Source: CAD feature listing. Evaluate the final solid. Frame: model axes, mm. A direction names the side the tool comes from. Round coordinates to 2 decimals unless told otherwise and drop trailing zeros. Loops run counter-clockwise (first coordinate to the right, second up) from the corner with the lowest first, then second, coordinate; pieces in that order, holes last. Notation, with made-up numbers: M 63,83 L 74,83 A8 cw 74,96 Z; hole C 0,10.5 d9. An arc over 180 degrees is marked long. One line per item, written item: value.
from build123d import *

# Parameters (mm, degrees)
SKETCH_1_R          = 31.5
EXTRUDE_1_DEPTH     = 8
SKETCH_1_3_R        = 3.25
CUT_EXTRUDE_1_DEPTH = 8
SKETCH_1_4_R        = 17
CUT_EXTRUDE_2_DEPTH = 6
EXTRUDE_2_DEPTH     = 4
SKETCH_4_W          = 50
SKETCH_4_H          = 8.5
EXTRUDE_3_DEPTH     = 95
SKETCH_5_R          = 3.1
CUT_EXTRUDE_3_DEPTH = 10
SKETCH_5_3_R        = 6.75
SKETCH_5_3_R_2      = 3.1
CUT_EXTRUDE_4_DEPTH = 4.3
EXTRUDE_4_DEPTH     = 8
SKETCH_1_8_R        = 17
CUT_EXTRUDE_5_DEPTH = 8


with BuildPart() as part:
    # Sketch 1 → Extrude 1 (new body)
    with BuildSketch(Plane.XY):
        Circle(SKETCH_1_R)
    extrude(amount=EXTRUDE_1_DEPTH)

    # Sketch 1_3 → Cut-Extrude 1 (cut)
    with BuildSketch(Plane.XY):
        with Locations((0, 25)):
            Circle(SKETCH_1_3_R)
        with Locations((-25, 0)):
            Circle(SKETCH_1_3_R)
        with Locations((25, 0)):
            Circle(SKETCH_1_3_R)
        with Locations((0, -25)):
            Circle(SKETCH_1_3_R)
    extrude(amount=CUT_EXTRUDE_1_DEPTH, mode=Mode.SUBTRACT)

    # Sketch 1_4 → Cut-Extrude 2 (cut)
    with BuildSketch(Plane.XY):
        Circle(SKETCH_1_4_R)
    extrude(amount=CUT_EXTRUDE_2_DEPTH, mode=Mode.SUBTRACT)

    # Sketch 1_5 → Extrude 2 (add)
    with BuildSketch(Plane.XY):
        with BuildLine():
            Line((25, 69.163767897), (17.863752341, 69.163767897))
            Line((17.863752341, 69.163767897), (-25, 69.163767897))
            Line((-25, 69.163767897), (-25, 28.735067362))
            Line((-25, 28.735067362), (-25, 19.163767897))
            ThreePointArc((-25, 19.163767897), (0, 31.5), (25, 19.163767897))
            Line((25, 19.163767897), (25, 69.163767897))
        make_face()
    extrude(amount=EXTRUDE_2_DEPTH)

    # Sketch 4 → Extrude 3 (add)
    with BuildSketch(Plane.XY.offset(4)):
        with Locations((0, 64.913767897)):
            Rectangle(SKETCH_4_W, SKETCH_4_H)
    extrude(amount=EXTRUDE_3_DEPTH)

    # Sketch 5 → Cut-Extrude 3 (cut)
    with BuildSketch(Plane.XZ.offset(-60.663767897)):
        with Locations(Location((0.088398714, 90, 0), (0, 0, 270))):
            Circle(SKETCH_5_R)
        with Locations(Location((0.088398714, 20, 0), (0, 0, 270))):
            Circle(SKETCH_5_R)
        with Locations(Location((0.088398714, 43.333, 0), (0, 0, 270))):
            Circle(SKETCH_5_R)
        with Locations(Location((0.088398714, 66.66667, 0), (0, 0, 270))):
            Circle(SKETCH_5_R)
    extrude(amount=-CUT_EXTRUDE_3_DEPTH, mode=Mode.SUBTRACT)

    # Sketch 5_3 → Cut-Extrude 4 (cut)
    # profile 1 of 4: a face of its own
    with BuildSketch(Plane.XZ.offset(-60.663767897)):
        with Locations(Location((0.088398714, 66.66667, 0), (0, 0, 270))):
            Circle(SKETCH_5_3_R)
        with Locations(Location((0.088398714, 66.66667, 0), (0, 0, 270))):
            Circle(SKETCH_5_3_R_2, mode=Mode.SUBTRACT)
    # profile 2 of 4: a face of its own
    with BuildSketch(Plane.XZ.offset(-60.663767897)):
        with Locations(Location((0.088398714, 43.333, 0), (0, 0, 270))):
            Circle(SKETCH_5_3_R)
        with Locations(Location((0.088398714, 43.333, 0), (0, 0, 270))):
            Circle(SKETCH_5_3_R_2, mode=Mode.SUBTRACT)
    # profile 3 of 4: a face of its own
    with BuildSketch(Plane.XZ.offset(-60.663767897)):
        with Locations(Location((0.088398714, 20, 0), (0, 0, 270))):
            Circle(SKETCH_5_3_R)
        with Locations(Location((0.088398714, 20, 0), (0, 0, 270))):
            Circle(SKETCH_5_3_R_2, mode=Mode.SUBTRACT)
    # profile 4 of 4: a face of its own
    with BuildSketch(Plane.XZ.offset(-60.663767897)):
        with Locations(Location((0.088398714, 90, 0), (0, 0, 270))):
            Circle(SKETCH_5_3_R)
    extrude(amount=-CUT_EXTRUDE_4_DEPTH, mode=Mode.SUBTRACT)

    # Sketch 1_7 → Extrude 4 (add)
    with BuildSketch(Plane.XY):
        with BuildLine():
            Line((25, 69.163767897), (17.863752341, 69.163767897))
            Line((17.863752341, 69.163767897), (-25, 69.163767897))
            Line((-25, 69.163767897), (-25, 28.735067362))
            Line((-25, 28.735067362), (-25, 19.163767897))
            ThreePointArc((-25, 19.163767897), (0, 31.5), (25, 19.163767897))
            Line((25, 19.163767897), (25, 69.163767897))
        make_face()
    extrude(amount=EXTRUDE_4_DEPTH)

    # Sketch 1_8 → Cut-Extrude 5 (cut)
    with BuildSketch(Plane.XY):
        Circle(SKETCH_1_8_R)
    extrude(amount=CUT_EXTRUDE_5_DEPTH, mode=Mode.SUBTRACT)


solid = part.part
1. Reachability of faces 1 (the face through (-1, 64.964, 40)), 2 (the face through (0, 69.164, 49)), 3 (the face through (25, 61, 38)) from +Z, -Z, +X, -X, +Y, -Y: full face, straight path, thin tool, end or side. Return the list, or none.
Report:
face 1: -Y
face 2: +Z, -Z, +X, -X, +Y
face 3: +Z, -Z, +X, +Y
2. Section query A-A (z = 20). Return the cut outline in (x, y), and give its area (3 significant figures).
Report:
outline: M -25,60.66 L -6.66,60.66 L -6.66,64.96 L -3.01,64.96 L -3.01,69.16 L -25,69.16 Z; M 3.19,64.96 L 6.84,64.96 L 6.84,60.66 L 25,60.66 L 25,69.16 L 3.19,69.16 Z
area: 341 mm2
3. Section query B-B (y = 25). Return the cut outline in (x, z), and give its area (3 significant figures).
Report:
outline: M -25,0 L -3.25,0 L -3.25,8 L -25,8 Z; M 3.25,0 L 25,0 L 25,8 L 3.25,8 Z
area: 348 mm2
4. Section query C-C (y = 1.5). Return the cut outline in (x, z), and give its area (3 significant figures).
Report:
outline: M -31.46,0 L -27.88,0 L -27.88,8 L -31.46,8 Z; M -22.12,0 L -16.93,0 L -16.93,8 L -22.12,8 Z; M 16.93,0 L 22.12,0 L 22.12,8 L 16.93,8 Z; M 27.88,0 L 31.46,0 L 31.46,8 L 27.88,8 Z
area: 140 mm2
5. Pull-direction query (Z, two-part tool) for faces 4 (the face through (7, 25, 8)), 5 (the face through (-3, 64.964, 65)), 6 (the face through (-25, 61, 38)); classes: released by +Z, released by -Z, zero draft, split by the parting line, or undercut.
Report:
face 4: released by +Z
face 5: undercut
face 6: zero draft
6. Section query D-D (z = 91). Return the cut outline in (x, y).
Report:
outline: M -25,60.66 L -6.59,60.66 L -6.59,64.96 L -2.85,64.96 L -2.85,69.16 L -25,69.16 Z; M 3.02,64.96 L 6.76,64.96 L 6.76,60.66 L 25,60.66 L 25,69.16 L 3.02,69.16 Z
7. Pin query (flat end, axial travel): pin 1 (7 mm diameter, centred on x = 0.09, z = 43.33, fed in from -Y); pin 2 (7.5 mm diameter, centred on x = -25, y = 0, fed in from +Z); pin 3 (11 mm diameter, centred on x = 2.5, z = 66.5, fed in from -Y). Return the tip coordinate at first contact, or that it passes through.
Report:
pin 1: stops at y = 64.96
pin 2: stops at z = 8
pin 3: stops at y = 60.66
8. Ray query, line 1 (X direction, y = 67.5, z = 90); line 2 (X direction, y = 63.15, z = 90); line 3 (Z direction, x = -19.5, y = 39). Return the intervals inside material, ascending. Write a range as [from, to].
Report:
line 1: x = [-25, -3.01], [3.19, 25]
line 2: x = [-25, -6.66], [6.84, 25]
line 3: z = [0, 8]
